The listing builds one solid part. Answer for the finished solid, in the listing's coordinates (mm). Round coordinates to 2 decimals unless told otherwise and drop trailing zeros. Loops run counter-clockwise (first coordinate to the right, second up) from the corner with the lowest first, then second, coordinate; pieces in that order, holes last. Notation, with made-up numbers: (64.5, 56.25) -> (97.5, 56.25) arc R19 cw to (97.5, 88.25) -> close; hole circle Ø8 at (82, -34.5). An arc over 180 degrees is marked (long way). Write each question's results on one line, items separated by ' | '. Start each with the question number.
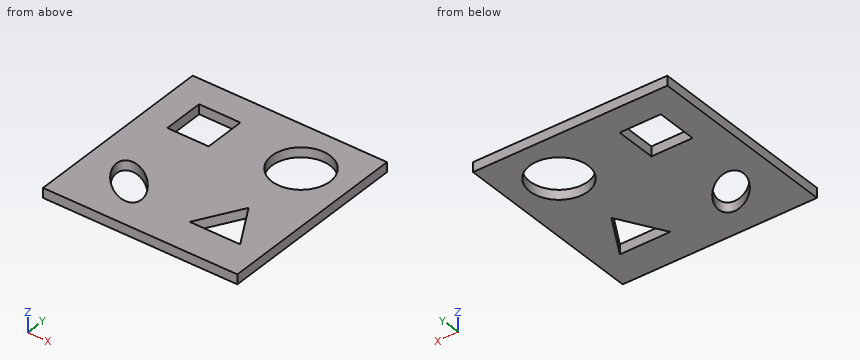
from build123d import *

# Parameters (mm, degrees)
SKETCH_W     = 200
SKETCH_H     = 200
PAD_DEPTH    = 10
SKETCH001_R  = 30
SKETCH001_W  = 42.426406
SKETCH001_H  = 42.426406
POCKET_DEPTH = 10.001


with BuildPart() as part:
    # Sketch → Pad (new body)
    with BuildSketch(Plane.XY):
        Rectangle(SKETCH_W, SKETCH_H)
    extrude(amount=PAD_DEPTH)

    # Sketch001 (on Face6 of Pad) → Pocket (cut, through all)
    with BuildSketch(Plane.XY.offset(10)):
        with Locations((50, 50)):
            Circle(SKETCH001_R)
        with BuildLine():
            add(Edge.make_bspline(
                [(-28.786797, -71.213203), (-10.415623, -52.84203), (-51.421015, -30.207812), (-92.426407, -7.573593), (-69.792188, -48.578985), (-47.15797, -89.584377), (-28.786797, -71.213203)],
                knots=[0, 0, 0, 2.094395, 2.094395, 4.18879, 4.18879, 6.283185, 6.283185, 6.283185], degree=2, weights=[1, 0.5, 1, 0.5, 1, 0.5, 1]))
        make_face()
        Polygon((75.980762, -65), (50, -20), (24.019238, -65), align=None)
        with Locations((-50, 50)):
            Rectangle(SKETCH001_W, SKETCH001_H)
    extrude(amount=-POCKET_DEPTH, mode=Mode.SUBTRACT)


solid = part.part
Item 1: The part is cut by section A-A, the plane y = 50. Give the vertices of the cut face in (x, z).
Item 2: The part is cut by section B-B, the plane z = 3.5. Give the number of separate pieces and of enclosed holes in the cut face, plus the area to 3 significant figures.
Item 3: Straight lines are drawn through the part: L1, parallel to Y at x = 50, z = 7.75; L2, parallel to Y at x = -61.5, z = 6; L3, parallel to X at y = -55, z = 5. For each, find the intervals that lie inside material, in ascending order. Write a range as [from, to].
Report:
1) outline: (-100, 0) -> (-71.21, 0) -> (-71.21, 10) -> (-100, 10) -> close; (-28.79, 0) -> (20, 0) -> (20, 10) -> (-28.79, 10) -> close; (80, 0) -> (100, 0) -> (100, 10) -> (80, 10) -> close
2) separate pieces: 1 | enclosed holes: 4 | area: 32,800 mm2
3) L1: y = [-100, -65], [-20, 20], [80, 100] | L2: y = [-100, -59.69], [-26.51, 28.79], [71.21, 100] | L3: x = [-100, -65.55], [-28.45, 29.79], [70.21, 100]
